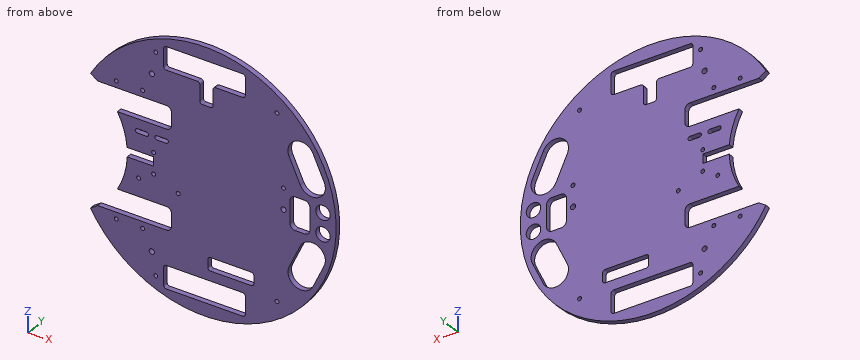
Autodesk Inventor part; units mm, degrees
ref_plane "YZ Plane" through (0, 0, 0) normal (1, 0, 0) x (0, 1, 0)
ref_plane "XZ Plane" through (0, 0, 0) normal (0, 1, 0) x (-1, 0, 0)
ref_plane "XY Plane" through (0, 0, 0) normal (0, 0, 1) x (1, 0, 0)
sketch "Skizze1" plane through (0, 0, 0) normal (0, 1, 0) x (-1, 0, 0)
  arc A0 (86.6025, 50) -> (86.6025, -50) centre (117.2454, 0) ccw
  arc A1 (86.6025, 50) -> (86.6025, -50) centre (0, 0) ccw
  line L0 (31, -90) -> (-31, -90)
  line L1 (-31, -90) -> (-31, -72.5)
  line L2 (-31, -72.5) -> (31, -72.5)
  line L3 (31, -72.5) -> (31, -90)
  line L4 (31, 72.5) -> (-31, 72.5)
  line L5 (-31, 72.5) -> (-31, 90)
  line L6 (-31, 90) -> (31, 90)
  line L7 (31, 90) -> (31, 72.5)
  circle A2 centre (67, -51.25) radius 1.5
  circle A3 centre (47, -51.25) radius 1.5
  circle A4 centre (67, 51.25) radius 1.5
  circle A5 centre (47, 51.25) radius 1.5
  line L8 (81.191, -46.25) -> (25, -46.25)
  line L9 (25, -46.25) -> (25, -28.75)
  line L10 (25, -28.75) -> (66.1335, -28.75)
  line L11 (66.1335, 28.75) -> (25, 28.75)
  line L12 (25, 28.75) -> (25, 46.25)
  line L13 (25, 46.25) -> (81.191, 46.25)
  circle A6 centre (38.6025, -8) radius 1.5
  circle A7 centre (38.6025, 8) radius 1.5
  line L14 (58.7952, 4.75) -> (38.6457, 4.75)
  line L15 (38.6457, 4.75) -> (38.6457, -2.25)
  line L16 (38.6457, -2.25) -> (58.6457, -2.25)
  line L17 (-80, -12.5) -> (-65, -12.5)
  line L18 (-65, -12.5) -> (-65, 12.5)
  line L19 (-65, 12.5) -> (-80, 12.5)
  line L20 (-80, 12.5) -> (-80, -12.5)
  circle A8 centre (50, -15) radius 1.5
  circle A9 centre (-55, -70) radius 1.5
  circle A10 centre (-55, 70) radius 1.5
  circle A11 centre (37, -83) radius 1.5
  circle A12 centre (37, 83) radius 1.5
  line L21 (-73.4, -45.0752) -> (-81.8, -26.9248) construction
  line L22 (-64.3248, -40.8752) -> (-72.7248, -22.7248)
  line L23 (-90.8752, -31.1248) -> (-82.4752, -49.2752)
  arc A13 (-82.4752, -49.2752) -> (-64.3248, -40.8752) centre (-73.4, -45.0752) ccw
  arc A14 (-72.7248, -22.7248) -> (-90.8752, -31.1248) centre (-81.8, -26.9248) ccw
  line L24 (-73.4, -45.0752) -> (-81.8, -26.9248) construction
  line L25 (-81.8, 26.9248) -> (-73.4, 45.0752) construction
  line L26 (-90.8752, 31.1248) -> (-82.4752, 49.2752)
  line L27 (-64.3248, 40.8752) -> (-72.7248, 22.7248)
  arc A15 (-90.8752, 31.1248) -> (-72.7248, 22.7248) centre (-81.8, 26.9248) ccw
  arc A16 (-64.3248, 40.8752) -> (-82.4752, 49.2752) centre (-73.4, 45.0752) ccw
  line L28 (-81.8, 26.9248) -> (-73.4, 45.0752) construction
  circle A17 centre (20, -16) radius 1.5
  circle A18 centre (-60, 16) radius 1.5
  line L29 (-2.5, -65) -> (-37.5, -65)
  line L30 (-37.5, -65) -> (-37.5, -55)
  line L31 (-37.5, -55) -> (-2.5, -55)
  line L32 (-2.5, -55) -> (-2.5, -65)
  circle A19 centre (-90, -8) radius 5.5
  circle A20 centre (-90, 8) radius 5.5
  line L33 (3.5, 72.5) -> (-6.5, 72.5)
  line L34 (-6.5, 72.5) -> (-6.5, 56.5)
  line L35 (-6.5, 56.5) -> (3.5, 56.5)
  line L36 (3.5, 56.5) -> (3.5, 72.5)
  line L37 (36, 19.75) -> (29, 19.75) construction
  line L38 (36, 21.35) -> (29, 21.35)
  line L39 (29, 18.15) -> (36, 18.15)
  arc A21 (36, 18.15) -> (36, 21.35) centre (36, 19.75) ccw
  arc A22 (29, 21.35) -> (29, 18.15) centre (29, 19.75) ccw
  line L40 (44, 19.75) -> (51, 19.75) construction
  line L41 (44, 21.35) -> (51, 21.35)
  line L42 (51, 18.15) -> (44, 18.15)
  arc A23 (44, 21.35) -> (44, 18.15) centre (44, 19.75) ccw
  arc A24 (51, 18.15) -> (51, 21.35) centre (51, 19.75) ccw
  circle A25 centre (40, -66) radius 2
  circle A26 centre (40, 66) radius 2
  circle A27 centre (-60, 0) radius 2
  point P0 (58.6025, 0)
  point P1 (-31, -81.25)
  point P2 (-31, 81.25)
  point P3 (-77.6, -36)
  point P4 (-77.6, -36)
  point P5 (-77.6, 36)
  point P6 (-77.6, 36)
  point P7 (32.5, 19.75)
  point P8 (47.5, 19.75)
  dimension "d1" = 100
  dimension "d3" = 28
  dimension "d11" = 17.5
  dimension "d12" = 17.5
  dimension "d13" = 72.5
  dimension "d14" = 72.5
  dimension "d15" = 62
  dimension "d16" = 62
  dimension "d17" = 31
  dimension "d18" = 3
  dimension "d19" = 3
  dimension "d20" = 3
  dimension "d21" = 3
  dimension "d22" = 20
  dimension "d23" = 20
  dimension "d25" = 17.5
  dimension "d26" = 17.5
  dimension "d27" = 46.25
  dimension "d28" = 46.25
  dimension "d31" = 5
  dimension "d32" = 5
  dimension "d33" = 25
  dimension "d34" = 47
  dimension "d35" = 3
  dimension "d36" = 3
  dimension "d37" = 16
  dimension "d38" = 8
  dimension "d39" = 20
  dimension "d50" = 7
  dimension "d51" = 47.75
  dimension "d52" = 20
  dimension "d53" = 15
  dimension "d54" = 25
  dimension "d55" = 12.5
  dimension "d57" = 65
  dimension "d100" = 3
  dimension "d101" = 3
  dimension "d102" = 3
  dimension "d103" = 3
  dimension "d104" = 3
  dimension "d105" = 70
  dimension "d106" = 70
  dimension "d107" = 55
  dimension "d108" = 83
  dimension "d109" = 83
  dimension "d110" = 37
  dimension "d111" = 50
  dimension "d112" = 15
  dimension "d113" = 20
  dimension "d114" = 20
  dimension "d115" = 10
  dimension "d117" = 10
  dimension "d119" = 77.6
  dimension "d120" = 73.4
  dimension "d121" = 36
  dimension "d122" = 36
  dimension "d125" = 16
  dimension "d126" = 20
  dimension "d127" = 3
  dimension "d128" = 3
  dimension "d129" = 80
  dimension "d130" = 32
  dimension "d132" = 10
  dimension "d133" = 35
extrude "Extrusion1" add sketch "Skizze1" along normal blind 4 contours A0 L13 L12 L11 L14 L15 L16 L10 L9 L8 A1
fillet "Rundung1" radius 4 8 edges at (65, 2, 12.5) (65, 2, -12.5) (80, 2, 12.5) (80, 2, -12.5) (-25, 2, -28.75) (-25, 2, -46.25) (-25, 2, 28.75) (-25, 2, 46.25)
fillet "Rundung2" radius 2 16 edges at (31, 2, 90) (31, 2, 72.5) (-31, 2, 72.5) (-31, 2, 90) (31, 2, -90) (31, 2, -72.5) (-31, 2, -90) (-31, 2, -72.5) (2.5, 2, -55) (37.5, 2, -55) (37.5, 2, -65) (2.5, 2, -65) (6.5, 2, 56.5) (-3.5, 2, 56.5) (-3.5, 2, 72.5) (6.5, 2, 72.5)
equation "\"d14\" = d13"
equation "\"d15\" = d16"
properties part number "middle panel"
Check sheet for the modelled part. Datum: model origin and axes. Units: mm. Round coordinates to 2 decimals unless told otherwise and drop trailing zeros. Loops run counter-clockwise (first coordinate to the right, second up) from the corner with the lowest first, then second, coordinate; pieces in that order, holes last. Notation, with made-up numbers: M 84.5,-9 L 92.5,-9 A33 ccw 92.5,30 Z; hole C 52,43 d2. An arc over 180 degrees is marked long. Answer as a JSON object with one key per item and string values.
1. Gauge pin test, flat ends, axial feed: P1, Ø1.5, axis at x = -66, y = 1.5, coming from the -Z side; P2, Ø2, axis at x = 26.5, y = 2, coming from the -Z side; P3, Ø2, axis at x = -49, y = 1, coming from the -Z side; P4, Ø5, axis at x = 60, z = 16, coming from the +Y side. Record the tip position at first contact, or that the pin passes through.
Reply:
{"P1": "stops at z = -75.78", "P2": "stops at z = -96.69", "P3": "stops at z = -87.73", "P4": "stops at y = 4"}
2. Scan lines: line 1 (Z direction, x = 60, y = 0.8); line 2 (Z direction, x = -20, y = 3.35); line 3 (Z direction, x = 13, y = 1.3). Record each from-to range of solid material in increasing order.
Reply:
{"line 1": "z = -80 to -2, 2 to 14.5, 17.5 to 80", "line 2": "z = -97.98 to -90, -72.5 to -17.5, -14.5 to 72.5, 90 to 97.98", "line 3": "z = -99.15 to -90, -72.5 to -65, -55 to 72.5, 90 to 99.15"}
3. Section check A-A (x = 17). Record the boundary of the cut face in (y, z), plus the area to 3 significant figures.
Reply:
{"outline": "M 0,-98.54 L 4,-98.54 L 4,-90 L 0,-90 Z; M 0,-72.5 L 4,-72.5 L 4,-65 L 0,-65 Z; M 0,-55 L 4,-55 L 4,72.5 L 0,72.5 Z; M 0,90 L 4,90 L 4,98.54 L 0,98.54 Z", "area": "608 mm²"}
4. Section check B-B (x = -11). Record the boundary of the cut face in (y, z).
Reply:
{"outline": "M 0,-99.39 L 4,-99.39 L 4,-90 L 0,-90 Z; M 0,-72.5 L 4,-72.5 L 4,72.5 L 0,72.5 Z; M 0,90 L 4,90 L 4,99.39 L 0,99.39 Z"}
5. Section check C-C (y = 0.8). State how many separate pieces and enclosed holes the cut face has, plus the area to 3 significant figures.
Reply:
{"separate pieces": "1", "enclosed holes": "26", "area": "21,900 mm²"}
